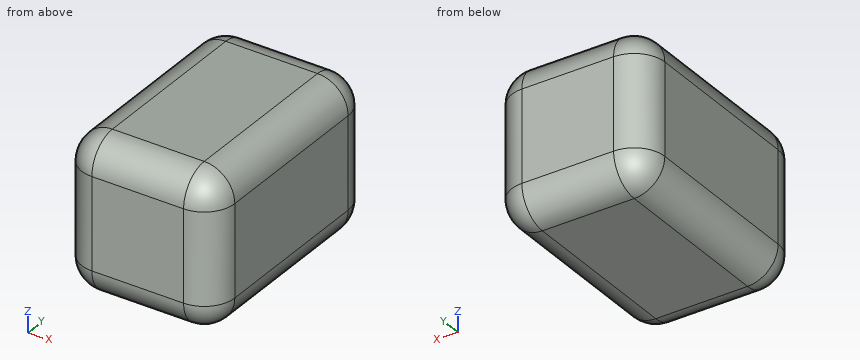
from build123d import *

# Parameters (mm, degrees)
F0_W     = 25.4
F0_H     = 38.1
F1_DEPTH = 25.4
F2_DEPTH = 25.4
F3_R     = 5.08
F4_R     = 5.08


with BuildPart() as f1:
    # F0 (on Top) → F1 (new body)
    with BuildSketch(Plane.XY):
        Rectangle(F0_W, F0_H)
    extrude(amount=F1_DEPTH)

    # F0 (on Top) → F2 (join)
    with BuildSketch(Plane.XY):
        Rectangle(F0_W, F0_H)
    extrude(amount=F2_DEPTH)

    # F3
    f3_edges = [f1.edges().sort_by_distance(p)[0] for p in [
        (-12.7, 0, 25.4),
        (12.7, 0, 25.4),
        (-12.7, 0, 0),
        (12.7, 0, 0),
    ]]
    fillet(f3_edges, radius=F3_R)

    # F4
    f4_edges = [f1.edges().sort_by_distance(p)[0] for p in [
        (0, -19.05, 25.4),
        (-12.7, -19.05, 12.7),
        (12.7, -19.05, 12.7),
        (-12.7, 19.05, 12.7),
        (12.7, 19.05, 12.7),
    ]]
    fillet(f4_edges, radius=F4_R)


solid = f1.part
Design review of the part built by this model. Coordinates are the model's own, in mm. Give positions to 0.01 mm unless a question says otherwise; leave off trailing zeros. Loops run counter-clockwise (first coordinate to the right, second up) from the corner with the lowest first, then second, coordinate; pieces in that order, holes last. Notation, with made-up numbers: (-35.5, 10) - (-7.5, 10) arc R14 ccw to (-7.5, 14) - close; hole circle Ø8 at (-37, 14.25). An arc over 180 degrees is marked (long way). Use CSV: the item, a comma, the result in double quotes. Start each with the question number.
1. Add section B-B (x = 4). State the section outline as (y, z) points, plus the area to 3 significant figures.
2. Wall thickness on L1, parallel to Y at x = -7.75, z = 17.75; L2, parallel to Z at x = -8.5, y = 11; L3, parallel to Y at x = 10.25, z = 13.25: over which ranges is each line inside the solid? List them lowest first.
3. Add section A-A (z = 15.5). State the section outline as (x, y) points.
4. Insertion check: P1, Ø1, axis at x = 9.5, z = 21.5, coming from the +Y side. The pin has a flat end and moves straight along its axis. Give the tip position at first contact, or say it passes through.
Results found:
1,outline,"(-19.05, 5.08) arc R5.08 ccw to (-13.97, 0) - (13.97, 0) arc R5.08 ccw to (19.05, 5.08) - (19.05, 20.32) arc R5.08 ccw to (13.97, 25.4) - (-13.97, 25.4) arc R5.08 ccw to (-19.05, 20.32) - close"
1,area,"946 mm²"
2,L1,"y = -19.05 to 19.05"
2,L2,"z = 0.08 to 25.32"
2,L3,"y = -18.32 to 18.32"
3,outline,"(-12.7, -13.97) arc R5.08 ccw to (-7.62, -19.05) - (7.62, -19.05) arc R5.08 ccw to (12.7, -13.97) - (12.7, 13.97) arc R5.08 ccw to (7.62, 19.05) - (-7.62, 19.05) arc R5.08 ccw to (-12.7, 13.97) - close"
4,P1,"stops at y = 18.75"
